Verification items for this drawing (mm, ordinates from the low corner). Coordinates: 2 decimals unless noted, no trailing zeros. Write each loop counter-clockwise with the first axis right and the second up, starting at its lowest first coordinate (ties: lowest second). Pieces come first, ordered by that corner, then holes.
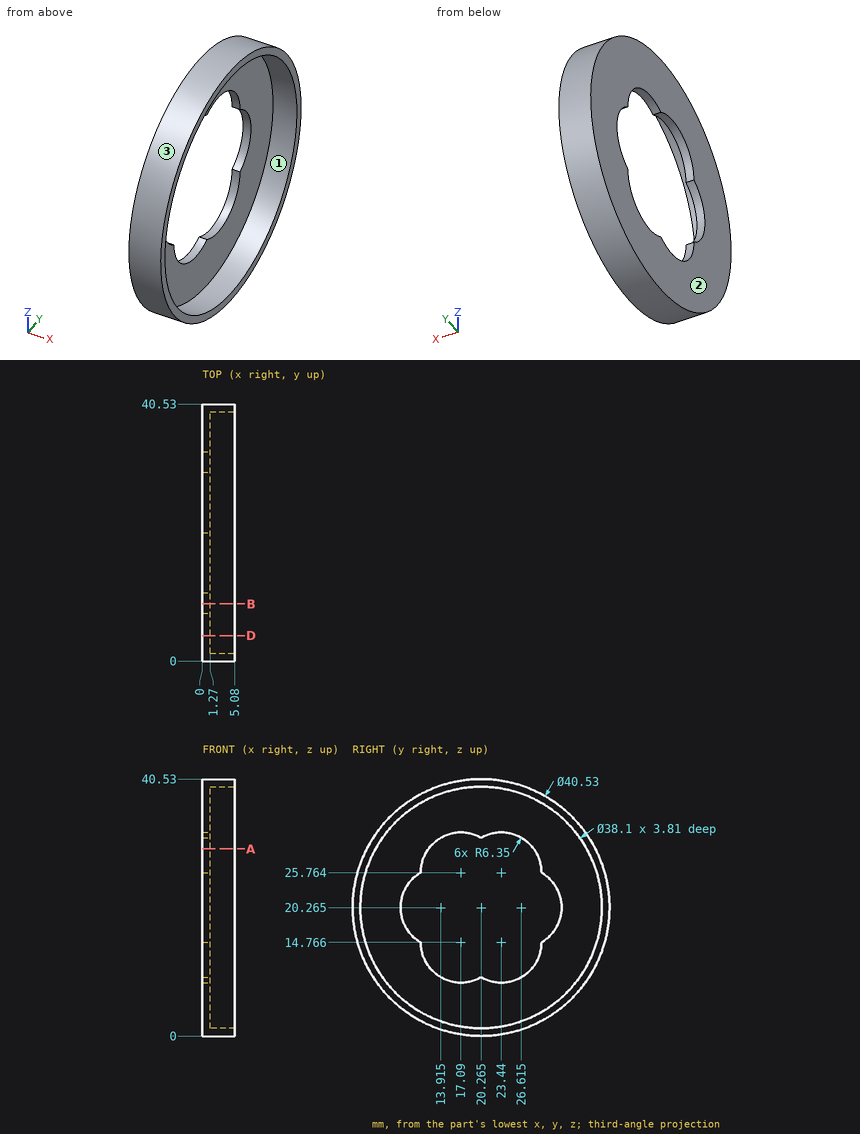
1. Sectioned sample at D-D, the plane y = 4. Record the boundary of the cut face in (x, z).
Computed values:
outline: (0, 8.18) - (5.08, 8.18) - (5.08, 10.35) - (1.27, 10.35) - (1.27, 30.18) - (5.08, 30.18) - (5.08, 32.35) - (0, 32.35) - close
2. Gauge pin test, flat ends, axial feed: pin 1 Ø1 at (x, z) = (3.5, 14.5) entering from -Y; pin 2 Ø1.5 at (x, y) = (1.5, 7) entering from -Z (1 decimal). Record the tip position at first contact, or that the pin passes through.
Computed values:
pin 1: stops at y = 0.7
pin 2: stops at z = 4.3
3. Draft check along Y on the marked faces 1, 2 and 3. Enter one of: released by +Y, released by -Y, zero draft, split by the parting line, or undercut.
Computed values:
face 1: undercut
face 2: zero draft
face 3: split by the parting line
4. Thickness scan on line 1 along Z through (x, y) = (2.6, 5) (1 decimal); line 2 along Y through (x, z) = (3.45, 6); line 3 along Z through (x, y) = (3.45, 36) (1 decimal). Record the ranges inside material, lowest first.
Computed values:
line 1: z = 6.9 to 8.9, 31.7 to 33.6
line 2: y = 5.87 to 7.64, 32.89 to 34.66
line 3: z = 7.5 to 9.5, 31 to 33
5. Sectioned sample at A-A, the plane z = 29.5. Record the boundary of the cut face in (x, y) (1 decimal).
Computed values:
outline: (0, 2.2) - (5.1, 2.2) - (5.1, 3.6) - (1.3, 3.6) - (1.3, 12) - (0, 12) - close; (0, 28.6) - (1.3, 28.6) - (1.3, 36.9) - (5.1, 36.9) - (5.1, 38.3) - (0, 38.3) - close
6. Sectioned sample at B-B, the plane y = 9. Record the boundary of the cut face in (x, z) (1 decimal).
Computed values:
outline: (0, 3.4) - (5.1, 3.4) - (5.1, 4.9) - (1.3, 4.9) - (1.3, 16.2) - (0, 16.2) - close; (0, 24.3) - (1.3, 24.3) - (1.3, 35.6) - (5.1, 35.6) - (5.1, 37.1) - (0, 37.1) - close
